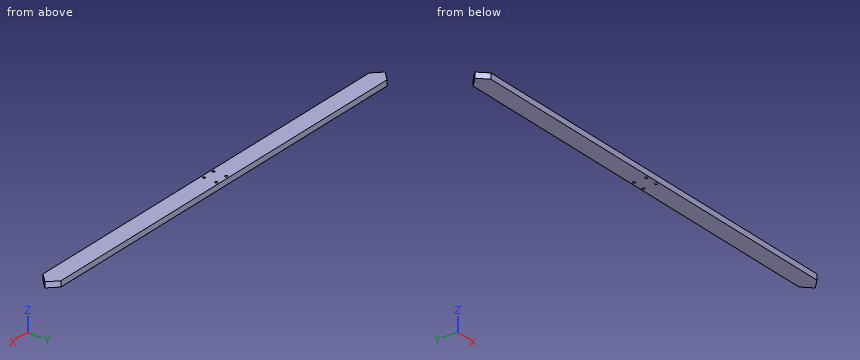
Autodesk Inventor part; units mm, degrees
ref_plane "YZ Plane" through (0, 0, 0) normal (1, 0, 0) x (0, 1, 0)
ref_plane "XZ Plane" through (0, 0, 0) normal (0, 1, 0) x (-1, 0, 0)
ref_plane "XY Plane" through (0, 0, 0) normal (0, 0, 1) x (1, 0, 0)
sketch "Sketch1" plane through (0, 0, 0) normal (0, 0, 1) x (1, 0, 0)
  line L0 (0, 0) -> (12.7, 12.7)
  line L1 (0, 0) -> (12.7, -12.7)
  line L2 (12.7, -12.7) -> (600.1258, -12.7)
  line L3 (600.1258, -12.7) -> (612.8258, 0)
  line L4 (612.8258, 0) -> (600.1258, 12.7)
  line L5 (600.1258, 12.7) -> (12.7, 12.7)
  line L6 (0, 0) -> (26.9875, 0) construction
  dimension "d0" = 90
  dimension "d1" = 45
  dimension "d2" = 612.8258
  dimension "d3" = 25.4
  dimension "d4" = 12.7
  dimension "d5" = 0
extrude "Extrusion1" add sketch "Sketch1" along normal blind 7.9375
sketch "Sketch2" plane through (0, 0, 7.9375) normal (0, 0, 1) x (1, 0, 0)
  line L0 (12.7, 12.7) -> (0, 0) construction
  line L1 (0, 0) -> (306.4129, 0) construction
  line L2 (600.1258, 12.7) -> (12.7, 12.7) construction
  line L3 (306.4129, 0) -> (306.4129, 138.1125) construction
  circle A0 centre (306.4129, 0) radius 12.5 construction
  line L4 (297.5741, 8.8388) -> (315.2517, 8.8388) construction
  line L5 (315.2517, 8.8388) -> (315.2517, -8.8388) construction
  line L6 (315.2517, -8.8388) -> (297.5741, -8.8388) construction
  line L7 (297.5741, -8.8388) -> (297.5741, 8.8388) construction
  circle A1 centre (297.5741, 8.8388) radius 1.75
  circle A2 centre (315.2517, 8.8388) radius 1.75
  circle A3 centre (315.2517, -8.8388) radius 1.75
  circle A4 centre (297.5741, -8.8388) radius 1.75
  dimension "d8" = 306.4129
  dimension "d9" = 25
  dimension "d10" = 3.5
  dimension "d11" = 3.5
  dimension "d12" = 3.5
  dimension "d13" = 3.5
extrude "Extrusion2" cut sketch "Sketch2" against normal through all
properties part number "Motor Strap 5-16"
Here's how the part is built. I have some questions about the finished solid (model axes, mm). Give positions to 0.01 mm unless a question says otherwise; leave off trailing zeros. Loops run counter-clockwise (first coordinate to the right, second up) from the corner with the lowest first, then second, coordinate; pieces in that order, holes last. Notation, with made-up numbers: (42.5, 61) -> (98.5, 61) arc R20 ccw to (98.5, 87) -> close; hole circle Ø9 at (-0.5, 55.25). An arc over 180 degrees is marked (long way). One line per item, written item: value.
Q1. Suppose I cut it at A-A on z = 5.75. Please give me the cut outline in (x, y), then the cut area to 3 significant figures.
Answers follow:
outline: (0, 0) -> (12.7, -12.7) -> (600.13, -12.7) -> (612.83, 0) -> (600.13, 12.7) -> (12.7, 12.7) -> close; hole circle Ø3.5 at (297.57, -8.84); hole circle Ø3.5 at (297.57, 8.84); hole circle Ø3.5 at (315.25, -8.84); hole circle Ø3.5 at (315.25, 8.84)
area: 15,200 mm^2
Q2. If I drill on line 1 along X through (y, z) = (-10.25, 4.25); line 2 along X through (y, z) = (0.5, 5); line 3 along X through (y, z) = (4, 4.25), over which ranges is the centre line in solid material (lowest first)?
Answers follow:
line 1: 10.25 to 296.54, 298.61 to 314.22, 316.29 to 602.58
line 2: 0.5 to 612.33
line 3: 4 to 608.83
Q3. I'm going to push flat-ended pins straight in: pin 1 Ø2 at (y, z) = (-5.5, 2.5) entering from -X; pin 2 Ø3 at (x, y) = (474.5, -9.5) entering from -Z. Where does each tip first touch, or does it pass through?
Answers follow:
pin 1: x = 4.5
pin 2: z = 0
